Geometry check sheet. Reference: the model listing, model coordinates, mm. A direction names the side the tool comes from. Round coordinates to 2 decimals unless told otherwise and drop trailing zeros. Order: outer loops, then holes, each group sorted by start corner. A loop starts at its lowest first (then second) coordinate and runs counter-clockwise, first axis right, second up. Notation, with made-up numbers: (86, 38.25) - (137, 38.25) arc R17 ccw to (137, 42.25) - close; hole circle Ø2 at (32, -16). An arc over 180 degrees is marked (long way). Use a Markdown table: item, result. Add a question column.
(1) Thickness scan on line 1 along X through (y, z) = (-13.5, -202); line 2 along Z through (x, y) = (744, 11.5); line 3 along Z through (x, y) = (1346, -37). Record the ranges inside material, lowest first. Write a range as [from, to].
(2) Gauge pin test, flat ends, axial feed: P1, Ø1, axis at x = 1529.5, y = 30, coming from the +Z side; P2, Ø18.5, axis at x = 812.8, y = 0, coming from the -Z side. Record the tip position at first contact, or that the pin passes through.
(3) Mould release check, pull along Y, two halves, no side actions. Record for faces 4 (the face through (893, 38.1, -10)), 5 (the face through (877, -1, 36.576)), 6 (the face through (877, -1, 38.1)): released by +Y, released by -Y, zero draft, split by the parting line, or undercut.
(4) Access from +Z, -Z, +X, -X, +Y, -Y to the whole of each face (thin tool, end or side, straight path). Record for faces 1 (the face through (1653.14, -0.02, -123.3)), 2 (the face through (3.048, -1, 1)), 3 (the face through (89, 1.524, -96)).
(5) Section check A-A on y = 24. Record the boundary of the cut face in (x, z).
```python
from build123d import *

# Parameters (mm, degrees)
F0_W       = 76.2
F0_H       = 76.2
F0_W_2     = 73.152
F0_H_2     = 73.152
F1_DEPTH   = 1778
F6_D       = 15.875
F6_ON_F5_D = 15.875
F8_DEPTH   = 1.524
F9_DEPTH   = 1.524
F10_W      = 76.2
F10_H      = 353.2152473927
F10_R      = 7.9375
F11_DEPTH  = 3.048


with BuildPart() as f1:
    # F0 (on Right) → F1 (new body)
    with BuildSketch(Plane.YZ):
        Rectangle(F0_W, F0_H)
        Rectangle(F0_W_2, F0_H_2, mode=Mode.SUBTRACT)
    extrude(amount=F1_DEPTH)

    # F6 (through all)
    with Locations(Plane.XZ.offset(76.2)):
        with Locations((76.2, 0), (127, 0), (177.8, 0), (228.6, 0), (279.4, 0), (330.2, 0), (381, 0), (431.8, 0), (482.6, 0), (533.4, 0), (584.2, 0), (635, 0), (685.8, 0), (736.6, 0), (787.4, 0), (838.2, 0), (889, 0), (939.8, 0), (990.6, 0), (1041.4, 0), (1092.2, 0), (1143, 0), (1193.8, 0), (1244.6, 0), (1295.4, 0), (1346.2, 0), (1397, 0), (1447.8, 0), (1498.6, 0), (1549.4, 0), (1600.2, 0), (1651, 0), (1701.8, 0)):
            Hole(F6_D / 2)

    # F6 on F5 (through all)
    with Locations(Plane.XY.offset(76.2)):
        with Locations((1422.4, 0), (1270, 0), (1117.6, 0), (965.2, 0), (812.8, 0), (660.4, 0), (508, 0), (355.6, 0)):
            Hole(F6_ON_F5_D / 2)

    # F7 (on Front) → F8 (join)
    with BuildSketch(Plane.XZ):
        with BuildLine():
            Line((228.6, -38.1), (0, -38.1))
            Line((0, -38.1), (0, -63.9625564218))
            ThreePointArc((0, -63.9625564218), (33.2066453993, -97.1692018211), (0, -130.3758472204))
            Line((0, -130.3758472204), (0, -190.5))
            Line((0, -190.5), (23.9939857274, -190.5))
            Line((23.9939857274, -190.5), (228.6, -54.1826970875))
            Line((228.6, -54.1826970875), (228.6, -38.1))
        make_face()
    extrude(amount=F8_DEPTH)

    # F7 (on Front) → F9 (join)
    with BuildSketch(Plane.XZ):
        with BuildLine():
            Line((228.6, -38.1), (0, -38.1))
            Line((0, -38.1), (0, -63.9625564218))
            ThreePointArc((0, -63.9625564218), (33.2066453993, -97.1692018211), (0, -130.3758472204))
            Line((0, -130.3758472204), (0, -190.5))
            Line((0, -190.5), (23.9939857274, -190.5))
            Line((23.9939857274, -190.5), (228.6, -54.1826970875))
            Line((228.6, -54.1826970875), (228.6, -38.1))
        make_face()
    extrude(amount=-F9_DEPTH)

    # F10 (on Right) → F11 (join)
    with BuildSketch(Plane.YZ):
        with Locations((0, -100.8058041334)):
            Rectangle(F10_W, F10_H)
        with Locations((0, -252.0134278297)):
            Circle(F10_R, mode=Mode.SUBTRACT)
        with Locations((0, -99.6134278297)):
            Circle(F10_R, mode=Mode.SUBTRACT)
        with Locations((0, 52.7865721703)):
            Circle(F10_R, mode=Mode.SUBTRACT)
    extrude(amount=F11_DEPTH)

    # F13: F1 across plane


with BuildPart() as f1_1:
    add(f1.part)
    add(f1.part.mirror(Plane.YZ.offset(889)))


solid = f1_1.part
```
Check sheet entries:
| question | item | result |
|---|---|---|
| 1 | line 1 | x = [0, 3.05], [1774.95, 1778] |
| 1 | line 2 | z = [-38.1, -36.58], [36.58, 38.1] |
| 1 | line 3 | z = [-38.1, -7.93], [7.93, 38.1] |
| 2 | P1 | stops at z = 38.1 |
| 2 | P2 | stops at z = -38.1 |
| 3 | face 4 | released by +Y |
| 3 | face 5 | undercut |
| 3 | face 6 | zero draft |
| 4 | face 1 | -Z, +Y, -Y |
| 4 | face 2 | none |
| 4 | face 3 | -Z, +Y |
| 5 | outline | (0, -277.41) - (3.05, -277.41) - (3.05, -38.1) - (1774.95, -38.1) - (1774.95, -277.41) - (1778, -277.41) - (1778, 75.8) - (1774.95, 75.8) - (1774.95, 38.1) - (3.05, 38.1) - (3.05, 75.8) - (0, 75.8) - close; hole (3.05, -36.58) - (1774.95, -36.58) - (1774.95, 36.58) - (3.05, 36.58) - close |
